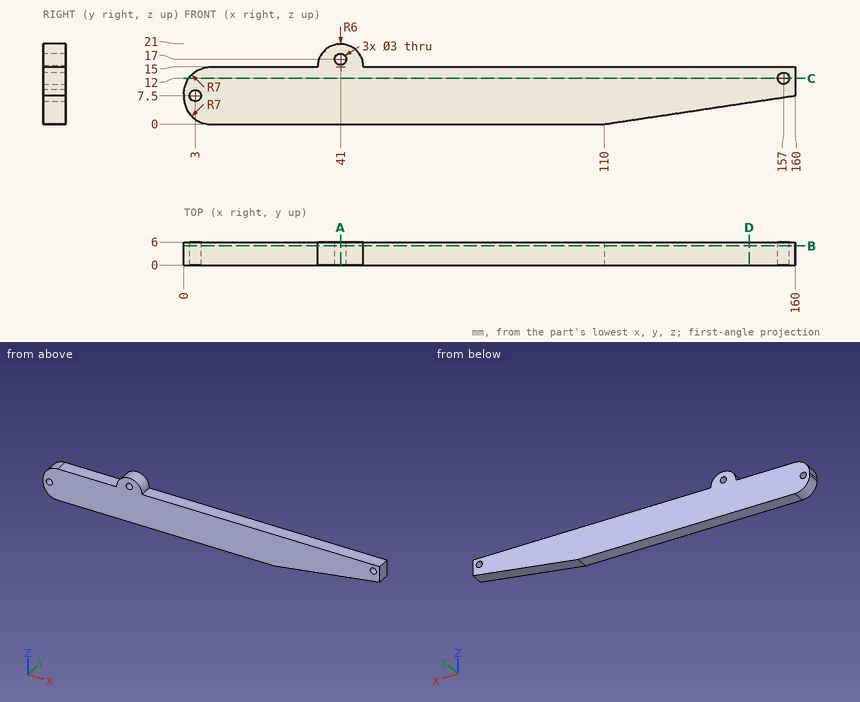
Here's the drawing with two shaded views (mm, measured from the low corner). I have some questions. Coordinates: 2 decimals unless noted, no trailing zeros. Loops run counter-clockwise (first coordinate to the right, second up) from the corner with the lowest first, then second, coordinate; pieces in that order, holes last. Notation, with made-up numbers: (3.25, 11) -> (22.25, 11) arc R17 ccw to (22.25, 31) -> close; hole circle Ø9 at (-36, 60.25). An arc over 180 degrees is marked (long way). Put each result on its own line as item: value. Start each with the question number.
Q1. I'm going to push flat-ended pins straight in: P1, Ø3, axis at y = 4.5, z = 18, coming from the -X side; P2, Ø4, axis at x = 41, z = 17, coming from the -Y side; P3, Ø1.8, axis at x = 89, y = 4.5, coming from the +Z side; P4, Ø3, axis at x = 34, y = 2.5, coming from the +Z side. Where does each tip first touch, or does it pass through?
Q2. I want a section at D-D (x = 148). Write out the boundary of the cut face in (y, z), plus the area to 3 significant figures.
Q3. I want a section at B-B (y = 5.05). Write out the boundary of the cut face in (x, z), plus the area to 3 significant figures.
Q4. I want a section at C-C (z = 12). Write out the boundary of the cut face in (x, y).
Q5. I want a section at A-A (x = 41). Write out the boundary of the cut face in (y, z).
Q6. If I drill on line 1 (Z direction, x = 41, y = 4.7); line 2 (Z direction, x = 91, y = 1.4); line 3 (X direction, y = 4.1, z = 12), over which ranges is the centre line in solid material (lowest first)? Write a range as [from, to].
Taken from the geometry:
1. P1: stops at x = 35.19
1. P2: stops at y = 0
1. P3: stops at z = 15
1. P4: stops at z = 17.4
2. outline: (0, 5.7) -> (6, 5.7) -> (6, 15) -> (0, 15) -> close
2. area: 55.8 mm2
3. outline: (0, 7) arc R7 ccw to (7, 0) -> (110, 0) -> (160, 7.5) -> (160, 15) -> (47, 15) arc R6 ccw to (35, 15) -> (7, 15) arc R7 ccw to (0, 8) -> close; hole circle Ø3 at (3, 7.5); hole circle Ø3 at (41, 17); hole circle Ø3 at (157, 12)
3. area: 2,230 mm2
4. outline: (1.26, 0) -> (155.5, 0) -> (155.5, 6) -> (1.26, 6) -> close; (158.5, 0) -> (160, 0) -> (160, 6) -> (158.5, 6) -> close
5. outline: (0, 0) -> (6, 0) -> (6, 15.5) -> (0, 15.5) -> close; (0, 18.5) -> (6, 18.5) -> (6, 21) -> (0, 21) -> close
6. line 1: z = [0, 15.5], [18.5, 21]
6. line 2: z = [0, 15]
6. line 3: x = [1.26, 155.5], [158.5, 160]
